Geometry check sheet. Reference: the model listing, model coordinates, mm. A direction names the side the tool comes from. Coordinates: 2 decimals unless noted, no trailing zeros. Loops run counter-clockwise (first coordinate to the right, second up) from the corner with the lowest first, then second, coordinate; pieces in that order, holes last.
from build123d import *

# Parameters (mm, degrees)
SKETCH_1_W          = 118
SKETCH_1_H          = 78
EXTRUDE_1_DEPTH     = 2
FILLET_1_R          = 4
EXTRUDE_START       = 16
EXTRUDE_4_DEPTH     = 16
EXTRUDE_5_DEPTH     = 9
SKETCH_6_R          = 2.5
CUT_EXTRUDE_1_DEPTH = 0.6
CUT_EXTRUDE_2_DEPTH = 2.1
CHAMFER_1_SIZE      = 4
EXTRUDE_6_DEPTH     = 7


with BuildPart() as part:
    # 草图1 → 凸台-拉伸1 (new body)
    with BuildSketch(Plane.XY):
        Rectangle(SKETCH_1_W, SKETCH_1_H)
    extrude(amount=EXTRUDE_1_DEPTH)

    # 圆角1
    fillet_1_edges = [part.edges().sort_by_distance(p)[0] for p in [
        (59, -39, 1),
        (-59, -39, 1),
        (-59, 39, 1),
        (59, 39, 1),
    ]]
    fillet(fillet_1_edges, radius=FILLET_1_R)

    # 草图4 → 凸台-拉伸4 (add)
    with BuildSketch(Plane.XY.offset(2).offset(EXTRUDE_START)):
        with BuildLine():
            Line((59, -35), (59, 35))
            ThreePointArc((59, 35), (57.828427125, 37.828427125), (55, 39))
            Line((55, 39), (-55, 39))
            ThreePointArc((-55, 39), (-57.828427125, 37.828427125), (-59, 35))
            Line((-59, 35), (-59, -35))
            ThreePointArc((-59, -35), (-57.828427125, -37.828427125), (-55, -39))
            Line((-55, -39), (55, -39))
            ThreePointArc((55, -39), (57.828427125, -37.828427125), (59, -35))
        make_face()
        with BuildLine():
            Line((57, -35), (57, 35))
            ThreePointArc((57, 35), (56.414213562, 36.414213562), (55, 37))
            Line((55, 37), (-55, 37))
            ThreePointArc((-55, 37), (-56.414213562, 36.414213562), (-57, 35))
            Line((-57, 35), (-57, -35))
            ThreePointArc((-57, -35), (-56.414213562, -36.414213562), (-55, -37))
            Line((-55, -37), (55, -37))
            ThreePointArc((55, -37), (56.414213562, -36.414213562), (57, -35))
        make_face(mode=Mode.SUBTRACT)
    extrude(amount=-EXTRUDE_4_DEPTH)

    # 草图5 → 凸台-拉伸5 (add)
    with BuildSketch(Plane.XY.offset(18)):
        with BuildLine():
            Line((-51, 35), (-51, 39))
            Line((-51, 39), (-55, 39))
            ThreePointArc((-55, 39), (-57.828427125, 37.828427125), (-59, 35))
            Line((-59, 35), (-59, 31))
            Line((-59, 31), (-55, 31))
            ThreePointArc((-55, 31), (-52.171572875, 32.171572875), (-51, 35))
        make_face()
        with BuildLine():
            Line((51, 39), (55, 39))
            ThreePointArc((55, 39), (57.828427125, 37.828427125), (59, 35))
            Line((59, 35), (59, 31))
            Line((59, 31), (55, 31))
            ThreePointArc((55, 31), (52.171572875, 32.171572875), (51, 35))
            Line((51, 35), (51, 39))
        make_face()
        with BuildLine():
            Line((51, -35), (51, -39))
            Line((51, -39), (55, -39))
            ThreePointArc((55, -39), (57.828427125, -37.828427125), (59, -35))
            Line((59, -35), (59, -31))
            Line((59, -31), (55, -31))
            ThreePointArc((55, -31), (52.171572875, -32.171572875), (51, -35))
        make_face()
        with BuildLine():
            Line((-51, -39), (-55, -39))
            ThreePointArc((-55, -39), (-57.828427125, -37.828427125), (-59, -35))
            Line((-59, -35), (-59, -31))
            Line((-59, -31), (-55, -31))
            ThreePointArc((-55, -31), (-52.171572875, -32.171572875), (-51, -35))
            Line((-51, -35), (-51, -39))
        make_face()
    extrude(amount=-EXTRUDE_5_DEPTH)

    # 草图6 → 切除-拉伸1 (cut)
    with BuildSketch(Plane.XY.offset(18)):
        with Locations((-55, 35)):
            Circle(SKETCH_6_R)
        with Locations(Location((55, 35, 0), (0, 0, 180))):
            Circle(SKETCH_6_R)
        with Locations((55, -35)):
            Circle(SKETCH_6_R)
        with Locations(Location((-55, -35, 0), (0, 0, 180))):
            Circle(SKETCH_6_R)
    extrude(amount=-CUT_EXTRUDE_1_DEPTH, mode=Mode.SUBTRACT)

    # 草图7 → 切除-拉伸2 (cut)
    with BuildSketch(Plane.XY.offset(17.4)):
        with BuildLine():
            Line((53.309526953, 38.625231148), (52.886908691, 39.531538935))
            ThreePointArc((52.886908691, 39.531538935), (58.535533906, 38.535533906), (59.531538935, 32.886908691))
            Line((59.531538935, 32.886908691), (58.625231148, 33.309526953))
            ThreePointArc((58.625231148, 33.309526953), (58.395478624, 33.940766826), (57.76423875, 33.711014302))
            ThreePointArc((57.76423875, 33.711014302), (52.843324317, 32.843324317), (53.711014302, 37.76423875))
            ThreePointArc((53.711014302, 37.76423875), (53.940766826, 38.395478624), (53.309526953, 38.625231148))
        make_face()
        with BuildLine():
            Line((-58.625231148, 33.309526953), (-59.531538935, 32.886908691))
            ThreePointArc((-59.531538935, 32.886908691), (-58.535533906, 38.535533906), (-52.886908691, 39.531538935))
            Line((-52.886908691, 39.531538935), (-53.309526953, 38.625231148))
            ThreePointArc((-53.309526953, 38.625231148), (-53.940766826, 38.395478624), (-53.711014302, 37.76423875))
            ThreePointArc((-53.711014302, 37.76423875), (-52.843324317, 32.843324317), (-57.76423875, 33.711014302))
            ThreePointArc((-57.76423875, 33.711014302), (-58.395478624, 33.940766826), (-58.625231148, 33.309526953))
        make_face()
        with BuildLine():
            Line((58.625231148, -33.309526953), (59.531538935, -32.886908691))
            ThreePointArc((59.531538935, -32.886908691), (58.535533906, -38.535533906), (52.886908691, -39.531538935))
            Line((52.886908691, -39.531538935), (53.309526953, -38.625231148))
            ThreePointArc((53.309526953, -38.625231148), (53.940766826, -38.395478624), (53.711014302, -37.76423875))
            ThreePointArc((53.711014302, -37.76423875), (52.843324317, -32.843324317), (57.76423875, -33.711014302))
            ThreePointArc((57.76423875, -33.711014302), (58.395478624, -33.940766826), (58.625231148, -33.309526953))
        make_face()
        with BuildLine():
            Line((-53.309526953, -38.625231148), (-52.886908691, -39.531538935))
            ThreePointArc((-52.886908691, -39.531538935), (-58.535533906, -38.535533906), (-59.531538935, -32.886908691))
            Line((-59.531538935, -32.886908691), (-58.625231148, -33.309526953))
            ThreePointArc((-58.625231148, -33.309526953), (-58.395478624, -33.940766826), (-57.76423875, -33.711014302))
            ThreePointArc((-57.76423875, -33.711014302), (-52.843324317, -32.843324317), (-53.711014302, -37.76423875))
            ThreePointArc((-53.711014302, -37.76423875), (-53.940766826, -38.395478624), (-53.309526953, -38.625231148))
        make_face()
    extrude(amount=-CUT_EXTRUDE_2_DEPTH, mode=Mode.SUBTRACT)

    # 倒角1
    chamfer_1_edges = [part.edges().sort_by_distance(p)[0] for p in [
        (-56, 31, 9),
        (-51, 36, 9),
        (-52.171572875, 32.171572875, 9),
        (51, 36, 9),
        (56, 31, 9),
        (52.171572875, 32.171572875, 9),
        (56, -31, 9),
        (51, -36, 9),
        (52.171572875, -32.171572875, 9),
        (-56, -31, 9),
        (-51, -36, 9),
        (-52.171572875, -32.171572875, 9),
    ]]
    chamfer(chamfer_1_edges, length=CHAMFER_1_SIZE - 0.0001)  # a hair under: the kernel refuses the full size

    # 草图8 → 凸台-拉伸6 (add)
    with BuildSketch(Plane(origin=(0, 0, 9), x_dir=(-1, 0, 0), z_dir=(0, 0, -1))):
        with BuildLine():
            Line((-55, -37), (-55, -35))
            Line((-55, -35), (-57, -35))
            ThreePointArc((-57, -35), (-56.414213562, -36.414213562), (-55, -37))
        make_face()
        with BuildLine():
            Line((57, -35), (55, -35))
            Line((55, -35), (55, -37))
            ThreePointArc((55, -37), (56.414213562, -36.414213562), (57, -35))
        make_face()
        with BuildLine():
            Line((55, 37), (55, 35))
            Line((55, 35), (57, 35))
            ThreePointArc((57, 35), (56.414213562, 36.414213562), (55, 37))
        make_face()
        with BuildLine():
            Line((-57, 35), (-55, 35))
            Line((-55, 35), (-55, 37))
            ThreePointArc((-55, 37), (-56.414213562, 36.414213562), (-57, 35))
        make_face()
    extrude(amount=EXTRUDE_6_DEPTH)


solid = part.part
1) Section check B-B on x = -46.5. Record the cut outline in (y, z).
Data:
outline: (-39, 0) - (39, 0) - (39, 18) - (37, 18) - (37, 2) - (-37, 2) - (-37, 18) - (-39, 18) - close
2) Section check C-C on y = -27.5. Record the cut outline in (x, z).
Data:
outline: (-59, 0) - (59, 0) - (59, 18) - (57, 18) - (57, 2) - (-57, 2) - (-57, 18) - (-59, 18) - close
3) Material ranges on probe 1 along Y at (x, z) = (-55, 17.85); probe 2 along X at (y, z) = (-35, 16.55); probe 3 along Y at (x, z) = (-7, 14.25), recorded low to high.
Data:
probe 1: y = -39 to -37.5, -32.5 to -31, 31 to 32.5, 37.5 to 39
probe 2: x = -51.95 to -51, 51 to 51.95
probe 3: y = -39 to -37, 37 to 39
4) Access from +Z, -Z, +X, -X, +Y, -Y to the whole of each face (thin tool, end or side, straight path). Record for faces 1 (the flat face through (-57, 37, 17.4)), 2 (the flat face through (-1, 1, 0)).
Data:
face 1: none
face 2: -Z, +X, -X, +Y, -Y
5) Depth check by flat-ended pin: pin 1 (1.6 mm diameter, centred on x = 56, z = 16, fed in from +Y); pin 2 (22 mm diameter, centred on x = -2.5, y = 0.5, fed in from +Z); pin 3 (0.6 mm diameter, centred on y = -35.5, z = 14.5, fed in from -X) (3 decimals). Enter the tip coordinate at first touch or a pass-through.
Data:
pin 1: stops at y = 38.95
pin 2: stops at z = 2
pin 3: stops at x = -58.995
6) Section check A-A on z = 4.75. Record the cut outline in (x, y).
Data:
outline: (-59, -35) arc R4 ccw to (-55, -39) - (55, -39) arc R4 ccw to (59, -35) - (59, 35) arc R4 ccw to (55, 39) - (-55, 39) arc R4 ccw to (-59, 35) - close; hole (-57, -35) - (-55, -35) - (-55, -37) - (55, -37) - (55, -35) - (57, -35) - (57, 35) - (55, 35) - (55, 37) - (-55, 37) - (-55, 35) - (-57, 35) - close
7) Mould release check, pull along Y, two halves, no side actions. Record for faces 3 (the flat face through (1, 37, 10)), 4 (the flat face through (59, 0, 9)), 5 (the cylindrical face through (-57.859, -37.797, 17.704)): +Y half, -Y half, draft (parallel to the pull), parting line (faces both ways), or undercut.
Data:
face 3: undercut
face 4: draft
face 5: -Y half
